from build123d import *

# Parameters (mm, degrees)
BOX003_W          = 10
BOX003_H          = 10
BOX003_DEPTH      = 2.7
BOX004_W          = 10
BOX004_H          = 10
BOX004_DEPTH      = 2.7
CYLINDER001_R     = 1.4
CYLINDER001_DEPTH = 10
CYLINDER_R        = 1.4
CYLINDER_DEPTH    = 10
BOX_W             = 30
BOX_H             = 1
BOX_DEPTH         = 8
BOX002_W          = 20
BOX002_H          = 5
BOX002_DEPTH      = 10
BOX001_W          = 30
BOX001_H          = 8
BOX001_DEPTH      = 2


with BuildPart() as obj1:
    # Box003 → Box003 (new body)
    with BuildSketch(Plane(origin=(17, 0, 3), x_dir=(1, 0, 0), z_dir=(0, 0, 1))):
        with Locations((5, 5)):
            Rectangle(BOX003_W, BOX003_H)
    extrude(amount=BOX003_DEPTH)


with BuildPart() as obj2:
    # Box004 → Box004 (new body)
    with BuildSketch(Plane(origin=(3, 0, 3), x_dir=(1, 0, 0), z_dir=(0, 0, 1))):
        with Locations((5, 5)):
            Rectangle(BOX004_W, BOX004_H)
    extrude(amount=BOX004_DEPTH)


with BuildPart() as zylinder001:
    # Cylinder001 → Cylinder001 (new body)
    with BuildSketch(Plane(origin=(27.5, 5.5, 0), x_dir=(1, 0, 0), z_dir=(0, 0, 1))):
        Circle(CYLINDER001_R)
    extrude(amount=CYLINDER001_DEPTH)


with BuildPart() as zylinder:
    # Cylinder → Cylinder (new body)
    with BuildSketch(Plane(origin=(2.5, 5.5, 0), x_dir=(1, 0, 0), z_dir=(0, 0, 1))):
        Circle(CYLINDER_R)
    extrude(amount=CYLINDER_DEPTH)


with BuildPart() as obj3:
    # Box → Box (new body)
    with BuildSketch(Plane.XY):
        with Locations((15, 0.5)):
            Rectangle(BOX_W, BOX_H)
    extrude(amount=BOX_DEPTH)


with BuildPart() as obj4:
    # Box002 → Box002 (new body)
    with BuildSketch(Plane(origin=(5, 3, 0), x_dir=(1, 0, 0), z_dir=(0, 0, 1))):
        with Locations((10, 2.5)):
            Rectangle(BOX002_W, BOX002_H)
    extrude(amount=BOX002_DEPTH)


with BuildPart() as cut004:
    # Box001 → Box001 (new body)
    with BuildSketch(Plane.XY):
        with Locations((15, 4)):
            Rectangle(BOX001_W, BOX001_H)
    extrude(amount=BOX001_DEPTH)

    # Cut: cut obj4
    add(obj4.part, mode=Mode.SUBTRACT)

    # Fusion: union obj3
    add(obj3.part)

    # Cut001: cut Zylinder
    add(zylinder.part, mode=Mode.SUBTRACT)

    # Cut002: cut Zylinder001
    add(zylinder001.part, mode=Mode.SUBTRACT)

    # Cut003: cut obj2
    add(obj2.part, mode=Mode.SUBTRACT)

    # Cut004: cut obj1
    add(obj1.part, mode=Mode.SUBTRACT)


solid = cut004.part
CAD build for the part. Positions are in the model's coordinates, mm. A direction names the side the tool comes from. Coordinates: 2 decimals unless noted, no trailing zeros. Write each loop counter-clockwise with the first axis right and the second up, starting at its lowest first coordinate (ties: lowest second). Pieces come first, ordered by that corner, then holes. Notation, with made-up numbers: (27.25, 1.25) - (46.25, 1.25) arc R18 cw to (46.25, 16.25) - close; hole circle Ø11 at (62, -6.5). An arc over 180 degrees is marked (long way). Use a Markdown table: item, result. Add a question column.
Item 1: Mould opens along Y. For faces 1 (the face through (26.47, 6.45, 0.99)), 2 (the face through (27, 8, 1)), 3 (the face through (15, 0, 4)), 4 (the face through (30, 2.5, 1.6)) say: pulls with the +Y half, pulls with the -Y half, needs draft (parallel to the pull), parting line crosses it, or undercut.
Item 2: Band-saw the part on C-C, the plane z = 1. Give the cut face in (x, y).
Item 3: Band-saw the part on A-A, the plane x = 2.5. Give the cut face in (y, z), and give its area (3 significant figures).
Item 4: Drill centre lines: L1, parallel to X at y = 5.5, z = 0.4; L2, parallel to Z at x = 26.5, y = 0.5; L3, parallel to Y at x = 27.5, z = 0.65. Where is each one in solid material? Low to high. Write a range as from..to.
Item 5: Flat gauge pins, fed straight in: pin 1 (1.5 mm diameter, centred on y = 5, z = 1.5, fed in from -X); pin 2 (3 mm diameter, centred on x = 9.5, z = 6, fed in from +Y). Where does each tip first touch, or does it go through?
Item 6: 3-axis set-ups, long thin cutter, end or side, ignore diameter. For faces 5 (the face through (25, 5, 1)), 6 (the face through (7.9, 0.5, 3)), 7 (the face through (11, 2, 2)): which of +Z, -Z, +X, -X, +Y, -Y reach the whole face in a straight line?
Item 7: Band-saw the part on D-D, the plane x = 15.25. Give the cut face in (y, z).
Item 8: Band-saw the part on B-B, the plane y = 5.5. Give the cut face in (x, z).
Numbers:
| question | item | result |
|---|---|---|
| 1 | face 1 | undercut |
| 1 | face 2 | pulls with the +Y half |
| 1 | face 3 | pulls with the -Y half |
| 1 | face 4 | needs draft |
| 2 | outline | (0, 0) - (30, 0) - (30, 8) - (25, 8) - (25, 3) - (5, 3) - (5, 8) - (0, 8) - close; hole circle Ø2.8 at (2.5, 5.5); hole circle Ø2.8 at (27.5, 5.5) |
| 3 | outline | (0, 0) - (4.1, 0) - (4.1, 2) - (1, 2) - (1, 8) - (0, 8) - close; (6.9, 0) - (8, 0) - (8, 2) - (6.9, 2) - close |
| 3 | area | 16.4 mm2 |
| 4 | L1 | 0..1.1, 3.9..5, 25..26.1, 28.9..30 |
| 4 | L2 | 0..3, 5.7..8 |
| 4 | L3 | 0..4.1, 6.9..8 |
| 5 | pin 1 | x = 0 |
| 5 | pin 2 | y = 1 |
| 6 | face 5 | +Z, -Z, +Y |
| 6 | face 6 | +Y, -Y |
| 6 | face 7 | +Z, +X, -X, +Y |
| 7 | outline | (0, 0) - (3, 0) - (3, 2) - (1, 2) - (1, 8) - (0, 8) - close |
| 8 | outline | (0, 0) - (1.1, 0) - (1.1, 2) - (0, 2) - close; (3.9, 0) - (5, 0) - (5, 2) - (3.9, 2) - close; (25, 0) - (26.1, 0) - (26.1, 2) - (25, 2) - close; (28.9, 0) - (30, 0) - (30, 2) - (28.9, 2) - close |
